```python
from build123d import *

# Parameters (mm, degrees)
SKETCH_1_W               = 40
SKETCH_1_H               = 40
EXTRUDE_1_DEPTH          = 10
SKETCH_7_R               = 2.575
CUT_EXTRUDE_2_DEPTH      = 3.15
PATTERN_CIRCULAR_1_COUNT = 2
PATTERN_CIRCULAR_1_ANGLE = 90
FILLET_2_R               = 5


with BuildPart() as part:
    # Эскиз1 → Бобышка-Вытянуть1 (new body)
    with BuildSketch(Plane(origin=(0, 0, 0), x_dir=(1, 0, 0), z_dir=(0, 1, 0))):
        Rectangle(SKETCH_1_W, SKETCH_1_H)
    extrude(amount=-EXTRUDE_1_DEPTH)

    # Эскиз7 → Вырез-Вытянуть2 (cut)
    with BuildSketch(Plane.ZY.offset(20)):
        with Locations((0, -5.199176943)):
            Circle(SKETCH_7_R)
        with BuildLine():
            Line((1.2875, -2.969161528), (0, -2.225823057))
            Line((0, -2.225823057), (-1.2875, -2.969161528))
            ThreePointArc((-1.2875, -2.969161528), (0, -2.624176943), (1.2875, -2.969161528))
        make_face()
    cut_extrude_2 = extrude(amount=-CUT_EXTRUDE_2_DEPTH, mode=Mode.SUBTRACT)

    # Круговой массив1: Вырез-Вытянуть2 ×2 about axis
    pattern_circular_1_axis = Axis((0, -10, 0), (0, -1, 0))
    for i in range(1, PATTERN_CIRCULAR_1_COUNT):
        add(cut_extrude_2.rotate(pattern_circular_1_axis, i * PATTERN_CIRCULAR_1_ANGLE / (PATTERN_CIRCULAR_1_COUNT - 1)), mode=Mode.SUBTRACT)

    # Скругление2
    fillet_2_edges = [part.edges().sort_by_distance(p)[0] for p in [
        (20, 0, 0),
        (0, 0, 20),
        (20, -5, 20),
    ]]
    fillet(fillet_2_edges, radius=FILLET_2_R)


solid = part.part
```
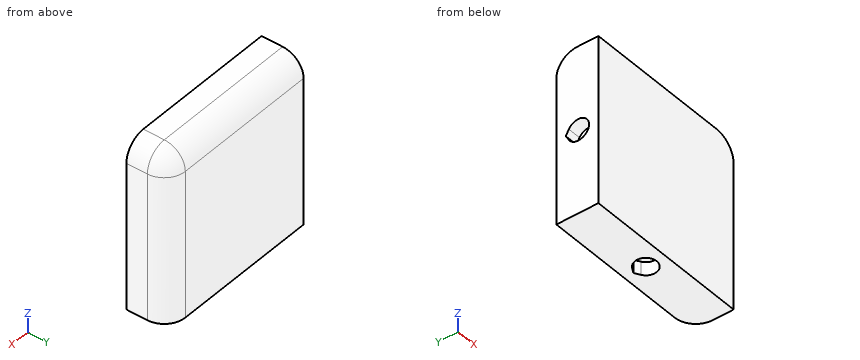
Input: part model. Units: mm. Frame: model coordinates. Coordinates: 2 decimals unless noted, no trailing zeros. Loops run counter-clockwise (first coordinate to the right, second up) from the corner with the lowest first, then second, coordinate; pieces in that order, holes last. Notation, with made-up numbers: M -13,-24 L 42,-24 A21 cw 42,-17 Z; hole C -37,45 d3. An arc over 180 degrees is marked long. One line per item, written item: value.
(1) Section A-A (y = -1). Output: boundary loops of the cut face in (x, z).
Filled in:
outline: M -20,-20 L 18,-20 L 18,15 A3 ccw 15,18 L -20,18 Z
(2) Section C-C (y = -5.5). Output: boundary loops of the cut face in (x, z).
Filled in:
outline: M -20,-20 L -2.56,-20 L -2.56,-16.85 L 2.56,-16.85 L 2.56,-20 L 20,-20 L 20,15 A5 ccw 15,20 L -20,20 L -20,2.56 L -16.85,2.56 L -16.85,-2.56 L -20,-2.56 Z
(3) Pin query (flat end, axial travel): pin 1 (1.5 mm diameter, centred on x = -0.5, y = -4.5, fed in from -Z). Return the tip coordinate at first contact, or that it passes through.
Filled in:
pin 1: z = -16.85
(4) Section B-B (z = 17). Output: boundary loops of the cut face in (x, y).
Filled in:
outline: M -20,-10 L 19.58,-10 L 19.58,-5 A4.58 ccw 15,-0.42 L -20,-0.42 Z
(5) Line query: line 1 along Y through (x, z) = (-18, 0); line 2 along Y through (x, z) = (17.5, 4.5); line 3 along Z through (x, y) = (17, -5.5). Output: solid intervals per line, ascending. Write a range as from..to.
Filled in:
line 1: -10..-7.77, -2.23..0
line 2: -10..-0.67
line 3: -20..19.58
